from build123d import *

# Parameters (mm, degrees)
SKETCH1_W           = 50.8
SKETCH1_H           = 22.86
BOSS_EXTRUDE1_DEPTH = 3.175
FILLET1_R           = 10.16
SKETCH3_R           = 1.651
CUT_EXTRUDE1_DEPTH  = 29.033649869
FILLET3_R           = 10.16
SKETCH4_W           = 34.036
SKETCH4_H           = 22.86
CUT_EXTRUDE2_DEPTH  = 29.033649869
FILLET4_R           = 3.175


with BuildPart() as part:
    # Sketch1 → Boss-Extrude1 (new body)
    with BuildSketch(Plane(origin=(0, 0, 0), x_dir=(1, 0, 0), z_dir=(0, 1, 0))):
        Rectangle(SKETCH1_W, SKETCH1_H)
    extrude(amount=BOSS_EXTRUDE1_DEPTH)

    # Fillet1
    fillet1_edges = [part.edges().sort_by_distance(p)[0] for p in [
        (25.4, 1.5875, 11.43),
        (-25.4, 1.5875, 11.43),
    ]]
    fillet(fillet1_edges, radius=FILLET1_R)

    # Sketch3 → Cut-Extrude1 (cut, through all)
    with BuildSketch(Plane(origin=(0, 3.175, 0), x_dir=(1, 0, 0), z_dir=(0, 1, 0))):
        with Locations(Location((15.24, -1.27, 0), (0, 0, 270))):
            Circle(SKETCH3_R)
        with Locations(Location((-3.81, -1.27, 0), (0, 0, 270))):
            Circle(SKETCH3_R)
    extrude(amount=-CUT_EXTRUDE1_DEPTH, mode=Mode.SUBTRACT)

    # Fillet3
    fillet3_edges = [part.edges().sort_by_distance(p)[0] for p in [
        (-25.4, 1.5875, -11.43),
        (25.4, 1.5875, -11.43),
    ]]
    fillet(fillet3_edges, radius=FILLET3_R)

    # Sketch4 → Cut-Extrude2 (cut, through all)
    with BuildSketch(Plane(origin=(0, 0, 0), x_dir=(-1, 0, 0), z_dir=(0, -1, 0))):
        with Locations((8.382, 0)):
            Rectangle(SKETCH4_W, SKETCH4_H)
    extrude(amount=-CUT_EXTRUDE2_DEPTH, mode=Mode.SUBTRACT)

    # Fillet4
    fillet4_edges = [part.edges().sort_by_distance(p)[0] for p in [
        (8.636, 1.5875, -11.43),
        (8.636, 1.5875, 11.43),
    ]]
    fillet(fillet4_edges, radius=FILLET4_R)


solid = part.part
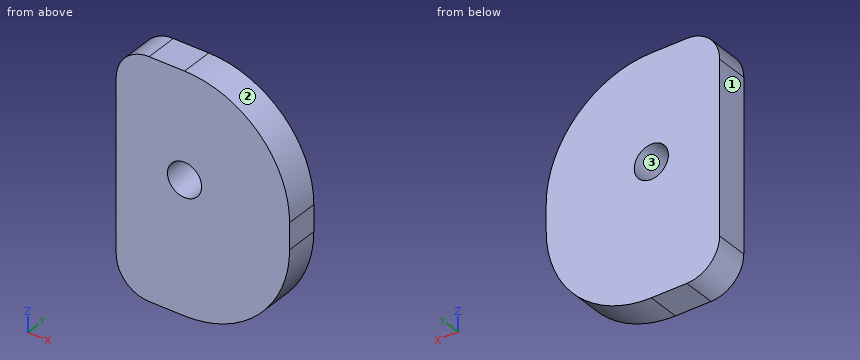
Read the model definition and answer for the solid it produces. Units are mm, in the model's axes. Face numbers are marked on the shaded views. Give positions to 0.01 mm unless a question says otherwise; leave off trailing zeros. Loops run counter-clockwise (first coordinate to the right, second up) from the corner with the lowest first, then second, coordinate; pieces in that order, holes last. Notation, with made-up numbers: (20.25, -15) - (59.25, -15) arc R13 ccw to (59.25, -6) - close; hole circle Ø11 at (-16.75, 9.5). An arc over 180 degrees is marked (long way). Answer as CSV lines item,"result". Start each with the question number.
1) Find section B-B (x = 19). Write down the section's boundary in (y, z) (3 decimals).
2) Find section A-A (y = 0.5). Write down the section's boundary in (x, z) (3 decimals), then the cut area to 3 significant figures.
3) This flat-tipped pin is pushed along its axis until it touches: pin 1 Ø1.5 at (y, z) = (1, 3) entering from +X. Where does it stop, or does it pass through?
4) Find section C-C (z = 8.75). Write down the section's boundary in (x, y) (3 decimals), then the cut area to 3 significant figures.
5) Straight lines are drawn through the part: L1, parallel to Z at x = 15, y = 1.45; L2, parallel to Z at x = 14.5, y = 2.75; L3, parallel to X at y = 1.1, z = 0.75. For each, find the intervals that lie inside material, in ascending order. Write a range as from..to.
6) Determine the mould class of the marked faces 1, 2 and 3 for opening direction Z: released by +Z, released by -Z, zero draft, split by the parting line, or undercut.
Findings below:
1,outline,"(0, -10.709) - (3.175, -10.709) - (3.175, 10.709) - (0, 10.709) - close"
2,outline,"(8.636, -8.255) arc R3.175 ccw to (11.811, -11.43) - (15.24, -11.43) arc R10.16 ccw to (25.4, -1.27) - (25.4, 1.27) arc R10.16 ccw to (15.24, 11.43) - (11.811, 11.43) arc R3.175 ccw to (8.636, 8.255) - close; hole circle Ø3.302 at (15.24, 1.27)"
2,area,"326 mm^2"
3,pin 1,"x = 25.35"
4,outline,"(8.675, 0) - (22.116, 0) - (22.116, 3.175) - (8.675, 3.175) - close"
4,area,"42.7 mm^2"
5,L1,"-11.43..-0.36, 2.9..11.43"
5,L2,"-11.43..-0.21, 2.75..11.43"
5,L3,"8.64..13.67, 16.81..25.4"
6,face 1,"zero draft"
6,face 2,"released by +Z"
6,face 3,"undercut"
